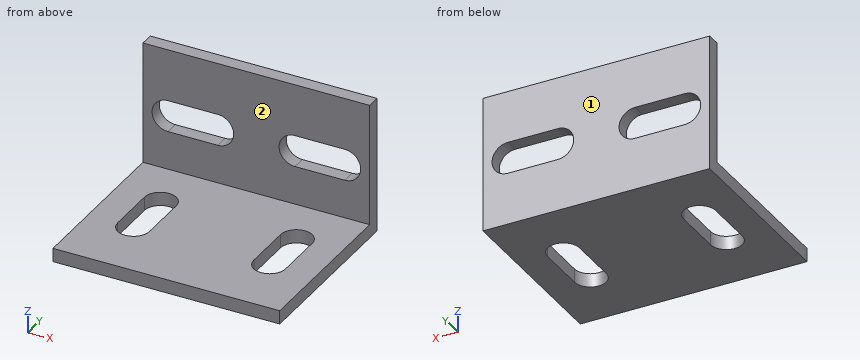
from build123d import *

# Parameters (mm, degrees)
F0_W     = 50
F0_H     = 40
F1_DEPTH = 3
F2_W     = 50
F2_H     = 3
F3_DEPTH = 27
F5_DEPTH = 3


with BuildPart() as f1:
    # F0 (on Top) → F1 (new body)
    with BuildSketch(Plane.XY):
        with Locations((0, 20)):
            Rectangle(F0_W, F0_H)
        with BuildLine():
            Line((-11.5, 25.5), (-11.5, 14.5))
            ThreePointArc((-11.5, 14.5), (-15, 11), (-18.5, 14.5))
            Line((-18.5, 14.5), (-18.5, 25.5))
            ThreePointArc((-18.5, 25.5), (-15, 29), (-11.5, 25.5))
        make_face(mode=Mode.SUBTRACT)
        with BuildLine():
            Line((11.5, 14.5), (11.5, 25.5))
            ThreePointArc((11.5, 25.5), (15, 29), (18.5, 25.5))
            Line((18.5, 25.5), (18.5, 14.5))
            ThreePointArc((18.5, 14.5), (15, 11), (11.5, 14.5))
        make_face(mode=Mode.SUBTRACT)
    extrude(amount=F1_DEPTH)

    # F2 (on face) → F3 (join)
    with BuildSketch(Plane.XY.offset(3)):
        with Locations((0, 38.5)):
            Rectangle(F2_W, F2_H)
    extrude(amount=F3_DEPTH)

    # F4 (on face) → F5 (cut)
    with BuildSketch(Plane.XZ.offset(-37)):
        with BuildLine():
            Line((-19.5, 11.5), (-8.5, 11.5))
            ThreePointArc((-8.5, 11.5), (-5, 15), (-8.5, 18.5))
            Line((-8.5, 18.5), (-19.5, 18.5))
            ThreePointArc((-19.5, 18.5), (-23, 15), (-19.5, 11.5))
        make_face()
        with BuildLine():
            ThreePointArc((8.5, 18.5), (5, 15), (8.5, 11.5))
            Line((8.5, 11.5), (19.5, 11.5))
            ThreePointArc((19.5, 11.5), (23, 15), (19.5, 18.5))
            Line((19.5, 18.5), (8.5, 18.5))
        make_face()
    extrude(amount=-F5_DEPTH, mode=Mode.SUBTRACT)


solid = f1.part
Geometry: final body of the model. Coordinates: model frame, mm. Face numbers are marked on the shaded views. A direction names the side the tool comes from. Give positions to 0.01 mm unless a question says otherwise; leave off trailing zeros. Write each loop counter-clockwise with the first axis right and the second up, starting at its lowest first coordinate (ties: lowest second). Pieces come first, ordered by that corner, then holes. Notation, with made-up numbers: (-0.75, 44) -> (15.25, 44) arc R18 ccw to (15.25, 72) -> close; hole circle Ø2 at (-1, 73.25). An arc over 180 degrees is marked (long way). Answer as a JSON object with one key per item and string values.
1. Contact query for flat-ended pins moving along their axis: pin 1 (2.5 mm diameter, centred on x = -12.5, y = 38, fed in from -Z); pin 2 (6 mm diameter, centred on x = 7, y = 32.5, fed in from +Z); pin 3 (4 mm diameter, centred on x = -12, z = 21, fed in from -Y). Output: stop coordinate, or through.
Ans:
{"pin 1": "stops at z = 0", "pin 2": "stops at z = 3", "pin 3": "stops at y = 37"}
2. Ray query, probe 1 along Z at (x, y) = (-17, 31.5); probe 2 along Y at (x, z) = (-3.5, 11.25); probe 3 along X at (y, z) = (38.5, 15.5). Return the intervals inside material, ascending. Write a range as from..to.
Ans:
{"probe 1": "z = 0..3", "probe 2": "y = 37..40", "probe 3": "x = -25..-22.96, -5.04..5.04, 22.96..25"}
3. Cut plane B-B on y = 23. Output: boundary loops of the cut face in (x, z).
Ans:
{"outline": "(-25, 0) -> (-18.5, 0) -> (-18.5, 3) -> (-25, 3) -> close; (-11.5, 0) -> (11.5, 0) -> (11.5, 3) -> (-11.5, 3) -> close; (18.5, 0) -> (25, 0) -> (25, 3) -> (18.5, 3) -> close"}
4. Cut plane C-C on x = 15. Output: boundary loops of the cut face in (y, z), and give its area (3 significant figures).
Ans:
{"outline": "(0, 0) -> (11, 0) -> (11, 3) -> (0, 3) -> close; (29, 0) -> (40, 0) -> (40, 11.5) -> (37, 11.5) -> (37, 3) -> (29, 3) -> close; (37, 18.5) -> (40, 18.5) -> (40, 30) -> (37, 30) -> close", "area": "126 mm^2"}
5. Cut plane A-A on z = 15. Output: boundary loops of the cut face in (x, y).
Ans:
{"outline": "(-25, 37) -> (-23, 37) -> (-23, 40) -> (-25, 40) -> close; (-5, 37) -> (5, 37) -> (5, 40) -> (-5, 40) -> close; (23, 37) -> (25, 37) -> (25, 40) -> (23, 40) -> close"}
6. Cut plane D-D on x = 7. Output: boundary loops of the cut face in (y, z).
Ans:
{"outline": "(0, 0) -> (40, 0) -> (40, 11.84) -> (37, 11.84) -> (37, 3) -> (0, 3) -> close; (37, 18.16) -> (40, 18.16) -> (40, 30) -> (37, 30) -> close"}
7. Access query for the marked faces 1 and 2. Directions: +Z, -Z, +X, -X, +Y, -Y. A direction counts if a zero-diameter tool reaches every point of the face in a straight line with its end or side. Return the directions, or none.
Ans:
{"face 1": "+Z, -Z, +X, -X, +Y", "face 2": "+Z, +X, -X, -Y"}
